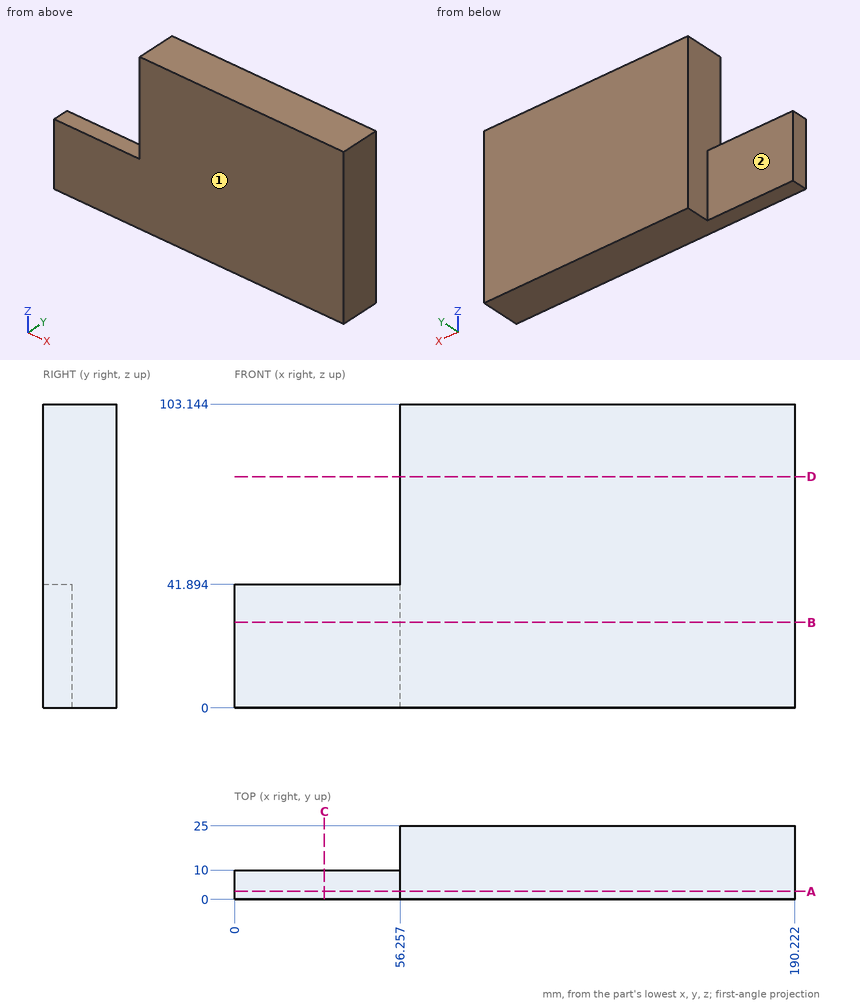
Input: dimensioned drawing with shaded views. Units: mm. Origin: part minimum x, y, z. A direction names the side the tool comes from. Coordinates: 2 decimals unless noted, no trailing zeros. Write each loop counter-clockwise with the first axis right and the second up, starting at its lowest first coordinate (ties: lowest second). Pieces come first, ordered by that corner, then holes. Notation, with made-up numbers: M 45.5,-3.5 L 72.5,-3.5 A33 ccw 72.5,24.5 Z; hole C 5,26.5 d7. An arc over 180 degrees is marked long. Answer as a JSON object with one key per item and string values. Group by question number.
(1) Contact query for flat-ended pins moving along their axis: P1, Ø10, axis at y = 18.5, z = 16, coming from the -X side; P2, Ø3, axis at x = 34.5, y = 4, coming from the +Z side; P3, Ø12.5, axis at x = 32, z = 27.5, coming from the +Y side. Output: stop coordinate, or through.
(2) Section B-B on z = 29. Output: boundary loops of the cut face in (x, y), plus the area to 3 significant figures.
(3) Section C-C on x = 30.5. Output: boundary loops of the cut face in (y, z).
(4) Set-up query: the marked faces 1 and 2. Return all of +Z, -Z, +X, -X, +Y, -Y with unobstructed straight access to the full face (end or side cutting, diameter ignored); none if empty.
(5) Section D-D on z = 78.5. Output: boundary loops of the cut face in (x, y).
(6) Section A-A on y = 2.75. Output: boundary loops of the cut face in (x, z) (1 decimal), plus the area to 3 significant figures.
(7) Ray query, line 1 along X through (y, z) = (14.75, 82.5); line 2 along Z through (x, y) = (13, 4.25); line 3 along Y through (x, z) = (40, 41.5). Return the intervals inside material, ascending. Write a range as [from, to].
Result set:
{
 "1": {"P1": "stops at x = 56.26", "P2": "stops at z = 41.89", "P3": "stops at y = 10"},
 "2": {"outline": "M 0,0 L 190.22,0 L 190.22,25 L 56.26,25 L 56.26,10 L 0,10 Z", "area": "3,910 mm2"},
 "3": {"outline": "M 0,0 L 10,0 L 10,41.89 L 0,41.89 Z"},
 "4": {"face 1": "+Z, -Z, +X, -X, -Y", "face 2": "+Z, -Z, -X, +Y"},
 "5": {"outline": "M 56.26,0 L 190.22,0 L 190.22,25 L 56.26,25 Z"},
 "6": {"outline": "M 0,0 L 190.2,0 L 190.2,103.1 L 56.3,103.1 L 56.3,41.9 L 0,41.9 Z", "area": "16,200 mm2"},
 "7": {"line 1": "x = [56.26, 190.22]", "line 2": "z = [0, 41.89]", "line 3": "y = [0, 10]"}
}
